The drawing under review shows one solid part. Ordinate dimensions are in mm from its lowest x, y, z. Give positions to 0.01 mm unless a question says otherwise; leave off trailing zeros. Loops run counter-clockwise (first coordinate to the right, second up) from the corner with the lowest first, then second, coordinate; pieces in that order, holes last. Notation, with made-up numbers: (-34, 32.25) -> (-11, 32.25) arc R13 ccw to (-11, 43.25) -> close; hole circle Ø4 at (46, -37.75). An arc over 180 degrees is marked (long way). Answer in a Markdown table with one row per item. Add a question column.
(1) Consider section C-C on z = 8. Write out the cut boundary in (x, y), then the cut area to 3 significant figures.
(2) Consider section A-A on y = 6.35. Write out the cut boundary in (x, z), then the cut area to 4 significant figures.
(3) For pin 1 (1 mm diameter, centred on y = 10.5, z = 8.5, fed in from +X); pin 2 (7.5 mm diameter, centred on x = 6.35, y = 6.35, fed in from -Z); pin 3 (1 mm diameter, centred on y = 7.5, z = 14.5, fed in from -X); pin 4 (5 mm diameter, centred on x = 6.35, y = 6.35, fed in from +Z), all flat-tipped, find the tip position at first contact; note any pin that passes through.
(4) Draft analysis for pull direction Y (two halves, no side actions). For the marked faces 1, 2 and 3, state which applies: +Y half, -Y half, draft (parallel to the pull), parting line (faces both ways), or undercut.
(5) For line 1 (X direction, y = 8.75, z = 13); line 2 (X direction, y = 8.5, z = 13.5); line 3 (Y direction, x = 7.25, z = 13.75), list the stretches that pass through material, from the lowest coordinate up.
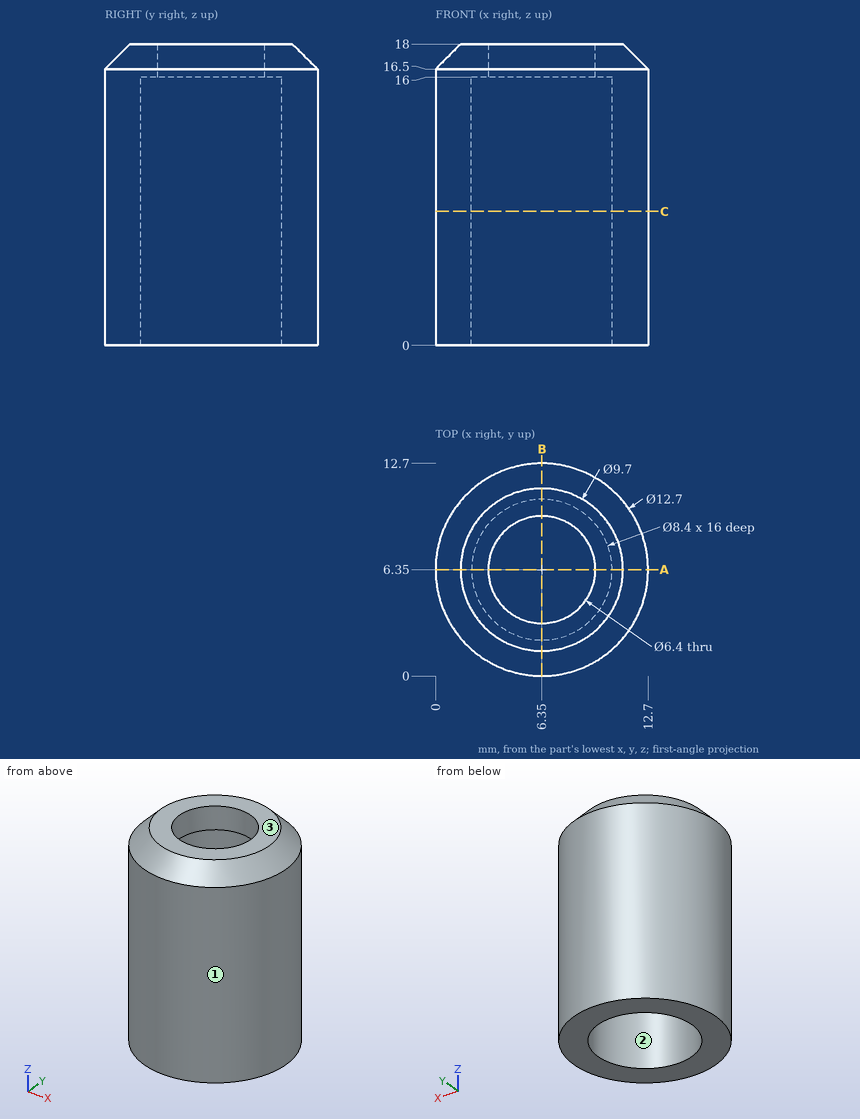
Values follow:
| question | item | result |
|---|---|---|
| 1 | outline | circle Ø12.7 at (6.35, 6.35); hole circle Ø8.4 at (6.35, 6.35) |
| 1 | area | 71.3 mm2 |
| 2 | outline | (0, 0) -> (2.15, 0) -> (2.15, 16) -> (3.15, 16) -> (3.15, 18) -> (1.5, 18) -> (0, 16.5) -> close; (9.55, 16) -> (10.55, 16) -> (10.55, 0) -> (12.7, 0) -> (12.7, 16.5) -> (11.2, 18) -> (9.55, 18) -> close |
| 2 | area | 79.15 mm2 |
| 3 | pin 1 | x = 11.55 |
| 3 | pin 2 | z = 16 |
| 3 | pin 3 | x = 0.03 |
| 3 | pin 4 | through |
| 4 | face 1 | parting line |
| 4 | face 2 | undercut |
| 4 | face 3 | draft |
| 5 | line 1 | 0.47 to 2.9, 9.8 to 12.23 |
| 5 | line 2 | 0.38 to 2.74, 9.96 to 12.32 |
| 5 | line 3 | 0.06 to 2.25, 10.45 to 12.64 |
